```python
from build123d import *

# Parameters (mm, degrees)
SKETCH_1_R                         = 5
SKETCH_1_R_2                       = 4
EXTRUDE_1_DEPTH                    = 16
SKETCH_2_R                         = 7.5
SKETCH_2_R_2                       = 5
EXTRUDE_2_DEPTH                    = 8.5
SKETCH_3_R                         = 10
SKETCH_3_R_2                       = 7.5
EXTRUDE_3_DEPTH                    = 12
SKETCH_4_R                         = 10
SKETCH_4_R_2                       = 2
EXTRUDE_4_DEPTH                    = 4.5
HOLE_WIZARD_M1_6_1_REACH           = 35.405
HOLE_WIZARD_M1_6_1_BORE_R          = 0.625
HOLE_WIZARD_M1_6_1_ON_FACE_2_REACH = 36.922
HOLE_WIZARD_M1_6_1_BORE_2_R        = 0.625


with BuildPart() as part:
    # 草图1 → 凸台-拉伸1 (new body)
    with BuildSketch(Plane(origin=(0, 0, 0), x_dir=(1, 0, 0), z_dir=(0, 1, 0))):
        with Locations(Location((0, 0, 0), (0, 0, 270))):
            Circle(SKETCH_1_R)
        with Locations(Location((0, 0, 0), (0, 0, 270))):
            Circle(SKETCH_1_R_2, mode=Mode.SUBTRACT)
    extrude(amount=EXTRUDE_1_DEPTH)

    # 草图2 → 凸台-拉伸2 (add)
    with BuildSketch(Plane.XZ):
        with Locations(Location((0, 0, 0), (0, 0, 270))):
            Circle(SKETCH_2_R)
        with Locations(Location((0, 0, 0), (0, 0, 270))):
            Circle(SKETCH_2_R_2, mode=Mode.SUBTRACT)
    extrude(amount=-EXTRUDE_2_DEPTH)

    # 草图3 → 凸台-拉伸3 (add)
    with BuildSketch(Plane.XZ):
        with Locations(Location((0, 0, 0), (0, 0, 270))):
            Circle(SKETCH_3_R)
        with Locations(Location((0, 0, 0), (0, 0, 270))):
            Circle(SKETCH_3_R_2, mode=Mode.SUBTRACT)
    extrude(amount=-EXTRUDE_3_DEPTH)

    # 草图4 → 凸台-拉伸4 (add)
    with BuildSketch(Plane.XZ):
        with BuildLine():
            Line((4.959164878, -20.878378378), (12.17249561, -5.837837838))
            ThreePointArc((12.17249561, -5.837837838), (13.5, 0), (12.17249561, 5.837837838))
            Line((12.17249561, 5.837837838), (4.959164878, 20.878378378))
            ThreePointArc((4.959164878, 20.878378378), (0, 24), (-4.959164878, 20.878378378))
            Line((-4.959164878, 20.878378378), (-12.17249561, 5.837837838))
            ThreePointArc((-12.17249561, 5.837837838), (-13.5, 0), (-12.17249561, -5.837837838))
            Line((-12.17249561, -5.837837838), (-4.959164878, -20.878378378))
            ThreePointArc((-4.959164878, -20.878378378), (0, -24), (4.959164878, -20.878378378))
        make_face()
        with Locations(Location((0, 0, 0), (0, 0, 270))):
            Circle(SKETCH_4_R, mode=Mode.SUBTRACT)
        with Locations(Location((0, 18.5, 0), (0, 0, 270))):
            Circle(SKETCH_4_R_2, mode=Mode.SUBTRACT)
        with Locations(Location((0, -18.5, 0), (0, 0, 270))):
            Circle(SKETCH_4_R_2, mode=Mode.SUBTRACT)
    extrude(amount=-EXTRUDE_4_DEPTH)

    # M1.6 螺纹孔1 bore (on position points) → M1.6 螺纹孔1 (cut, up to next)
    with BuildSketch(Plane(origin=(4.998978572, 13.886776662, -0.101060544), x_dir=(0.020212108711, 0, 0.999795714464), z_dir=(0.999795714464, 0, -0.020212108711)), mode=Mode.PRIVATE) as hole_wizard_m1_6_1_sk1:
        Circle(HOLE_WIZARD_M1_6_1_BORE_R)
    hole_wizard_m1_6_1_tool1 = extrude(hole_wizard_m1_6_1_sk1.sketch, amount=-HOLE_WIZARD_M1_6_1_REACH, mode=Mode.PRIVATE) & part.part
    add(hole_wizard_m1_6_1_tool1.solids().sort_by_distance((4.998979, 13.886777, -0.101061))[0], mode=Mode.SUBTRACT)

    # M1.6 螺纹孔1 bore 2 (on position points) → M1.6 螺纹孔1 on face 2 (cut, up to next)
    with BuildSketch(Plane(origin=(-0.028423278, 13.983100373, -4.999919211), x_dir=(-0.999983840262, 0, 0.005684999092), z_dir=(-0.005684999092, 0, -0.999983840262)), mode=Mode.PRIVATE) as hole_wizard_m1_6_1_on_face_2_sk1:
        Circle(HOLE_WIZARD_M1_6_1_BORE_2_R)
    hole_wizard_m1_6_1_on_face_2_tool1 = extrude(hole_wizard_m1_6_1_on_face_2_sk1.sketch, amount=-HOLE_WIZARD_M1_6_1_ON_FACE_2_REACH, mode=Mode.PRIVATE) & part.part
    add(hole_wizard_m1_6_1_on_face_2_tool1.solids().sort_by_distance((-0.028423, 13.9831, -4.999919))[0], mode=Mode.SUBTRACT)


solid = part.part
```
CAD build for the part. Positions are in the model's coordinates, mm. A direction names the side the tool comes from. Coordinates: 2 decimals unless noted, no trailing zeros. Order: outer loops, then holes, each group sorted by start corner. A loop starts at its lowest first (then second) coordinate and runs counter-clockwise, first axis right, second up.
(1) Saw through at C-C, the plane y = 6.5. Write the cut outline in (x, z).
Solution:
outline: circle Ø20 at (0, 0); hole circle Ø8 at (0, 0)
(2) Which spindle directions (+Z, -Z, +X, -X, +Y, -Y) get a long thin tool onto all of the face, cutting with end or side? Do faces 5 (the face through (9, 4.5, 6)), 6 (the face through (-8.616, 2.218, -13.253)). Say none if no direction does.
Solution:
face 5: +Y
face 6: -Z, -X, +Y, -Y
(3) Saw through at B-B, the plane z = 19. Write the cut outline in (x, y), and give its area (3 significant figures).
Solution:
outline: (-5.86, 0) - (-1.94, 0) - (-1.94, 4.5) - (-5.86, 4.5) - close; (1.94, 0) - (5.86, 0) - (5.86, 4.5) - (1.94, 4.5) - close
area: 35.3 mm2
(4) Mould opens along Z. For faces 1 (the face through (7, 12, -4)), 2 (the face through (-4.436, 12.198, 2.307)), 3 (the face through (13.5, 2.2, -0.1)), 4 (the face through (-8.515, 2.218, 13.463)) say: released by +Z, released by -Z, zero draft, split by the parting line, or undercut.
Solution:
face 1: zero draft
face 2: undercut
face 3: split by the parting line
face 4: released by +Z
(5) Saw through at A-A, the plane y = 2. Write the cut outline in (x, z), and give its area (3 significant figures).
Solution:
outline: (-12.17, -5.84) - (-4.96, -20.88) arc R5.5 ccw to (4.96, -20.88) - (12.17, -5.84) arc R13.5 ccw to (12.17, 5.84) - (4.96, 20.88) arc R5.5 ccw to (-4.96, 20.88) - (-12.17, 5.84) arc R13.5 ccw to start; hole circle Ø8 at (0, 0); hole circle Ø4 at (0, -18.5); hole circle Ø4 at (0, 18.5)
area: 789 mm2
(6) Saw through at D-D, the plane x = -9.5. Write the cut outline in (y, z).
Solution:
outline: (0, -11.41) - (4.5, -11.41) - (4.5, -3.12) - (12, -3.12) - (12, 3.12) - (4.5, 3.12) - (4.5, 11.41) - (0, 11.41) - close
(7) Pin check, flat tips, straight feed: pin 1 Ø3 at (x, y) = (2.5, 3) entering from -Z; pin 2 Ø13.5 at (x, z) = (0, 0) entering from +Y; pin 3 Ø4 at (x, z) = (-2.5, -18) entering from +Y; pin 4 Ø5 at (x, y) = (3.5, 10) entering from -Z. Stop position of each tip, or through.
Solution:
pin 1: stops at z = -23.91
pin 2: stops at y = 16
pin 3: stops at y = 4.5
pin 4: stops at z = -9.95
(8) Drill centre lines: L1, parallel to X at y = 10.4, z = 0; L2, parallel to Y at x = 4.25, z = 13.5; L3, parallel to Y at x = -3.5, z = -8. Where is each one in solid material? Low to high.
Solution:
L1: x = -10 to -7.5, -5 to -4, 4 to 5, 7.5 to 10
L2: y = 0 to 4.5
L3: y = 0 to 12
